from build123d import *

# Parameters (mm, degrees)
SKETCH1_R           = 25
SKETCH1_W           = 5
SKETCH1_H           = 10
SKETCH1_W_2         = 6
SKETCH1_H_2         = 8
BOSS_EXTRUDE1_DEPTH = 5


with BuildPart() as part:
    # Sketch1 → Boss-Extrude1 (new body)
    with BuildSketch(Plane.XY):
        with BuildLine():
            Line((-85, 10), (-85, 55))
            ThreePointArc((-85, 55), (-82.071067812, 62.071067812), (-75, 65))
            Line((-75, 65), (75, 65))
            ThreePointArc((75, 65), (82.071067812, 62.071067812), (85, 55))
            Line((85, 55), (85, 10))
            ThreePointArc((85, 10), (82.071067812, 2.928932188), (75, 0))
            Line((75, 0), (70, 0))
            ThreePointArc((70, 0), (40, -30), (10, 0))
            ThreePointArc((10, 0), (0, 10), (-10, 0))
            ThreePointArc((-10, 0), (-40, -30), (-70, 0))
            Line((-70, 0), (-75, 0))
            ThreePointArc((-75, 0), (-82.071067812, 2.928932188), (-85, 10))
        make_face()
        with Locations((-40, 0)):
            Circle(SKETCH1_R, mode=Mode.SUBTRACT)
        with Locations((40, 0)):
            Circle(SKETCH1_R, mode=Mode.SUBTRACT)
        with Locations((77.5, 17.5)):
            Rectangle(SKETCH1_W, SKETCH1_H, mode=Mode.SUBTRACT)
        with Locations((-77.5, 17.5)):
            Rectangle(SKETCH1_W, SKETCH1_H, mode=Mode.SUBTRACT)
        with Locations((-43, 42.5)):
            Rectangle(SKETCH1_W_2, SKETCH1_H_2, mode=Mode.SUBTRACT)
        with Locations((43, 42.5)):
            Rectangle(SKETCH1_W_2, SKETCH1_H_2, mode=Mode.SUBTRACT)
    extrude(amount=BOSS_EXTRUDE1_DEPTH)


solid = part.part
Geometry check sheet. Reference: the model listing, model coordinates, mm. A direction names the side the tool comes from. Round coordinates to 2 decimals unless told otherwise and drop trailing zeros. Order: outer loops, then holes, each group sorted by start corner. A loop starts at its lowest first (then second) coordinate and runs counter-clockwise, first axis right, second up. Notation, with made-up numbers: M 60,2 L 83,2 A17 ccw 83,25 Z; hole C -1,-5 d11. An arc over 180 degrees is marked long. Answer in a Markdown table with one row per item. Add a question column.
Item 1: Material ranges on L1, parallel to X at y = 45, z = 4.2; L2, parallel to X at y = -6, z = 4.6; L3, parallel to X at y = 1, z = 2.95, recorded low to high. Write a range as [from, to].
Item 2: Sectioned sample at A-A, the plane z = 3.25. State how many separate pieces and enclosed holes the cut face has, plus the area to 3 significant figures.
Item 3: Sectioned sample at C-C, the plane x = -60. Enter the section's corners in (y, z), plus the area to 3 significant figures.
Item 4: Depth check by flat-ended pin: pin 1 Ø2 at (x, z) = (-35.5, 4) entering from -Y; pin 2 Ø5 at (x, y) = (-66.5, -19) entering from -Z; pin 3 Ø2.5 at (x, z) = (76.5, 1.5) entering from -Y; pin 4 Ø1.5 at (x, z) = (-77.5, 2) entering from +Y. Enter the tip coordinate at first touch or a pass-through.
Item 5: Draft check along X on faces 3 (the face through (-82.15, 61.99, 2.46)), 4 (the face through (-1, 65, 2)), 5 (the face through (-80, 17, 2)). Enter one of: released by +X, released by -X, zero draft, split by the parting line, or undercut.
Item 6: Sectioned sample at D-D, the plane y = -11.5. Enter the section's corners in (x, z).
Item 7: Sectioned sample at B-B, the plane y = -23. Enter the section's corners in (x, z), plus the area to 3 significant figures.
Item 8: Set-up check for faces 1 (the face through (40.66, -29.993, 2.465)), 2 (the face through (75, 17, 2)): record each of +Z, -Z, +X, -X, +Y, -Y from which the full face is reachable in a straight line by a thin tool's end or side.
Filled in:
| question | item | result |
|---|---|---|
| 1 | L1 | x = [-85, -46], [-40, 40], [46, 85] |
| 1 | L2 | x = [-69.39, -64.27], [-15.73, -10.61], [10.61, 15.73], [64.27, 69.39] |
| 1 | L3 | x = [-79.36, -64.98], [-15.02, -9.95], [9.95, 15.02], [64.98, 79.36] |
| 2 | separate pieces | 1 |
| 2 | enclosed holes | 6 |
| 2 | area | 9,510 mm² |
| 3 | outline | M -22.36,0 L -15,0 L -15,5 L -22.36,5 Z; M 15,0 L 65,0 L 65,5 L 15,5 Z |
| 3 | area | 287 mm² |
| 4 | pin 1 | stops at y = -29.8 |
| 4 | pin 2 | passes through |
| 4 | pin 3 | stops at y = 0 |
| 4 | pin 4 | stops at y = 64.85 |
| 5 | face 3 | released by -X |
| 5 | face 4 | zero draft |
| 5 | face 5 | undercut |
| 6 | outline | M -67.71,0 L -62.2,0 L -62.2,5 L -67.71,5 Z; M -17.8,0 L -12.29,0 L -12.29,5 L -17.8,5 Z; M 12.29,0 L 17.8,0 L 17.8,5 L 12.29,5 Z; M 62.2,0 L 67.71,0 L 67.71,5 L 62.2,5 Z |
| 7 | outline | M -59.26,0 L -49.8,0 L -49.8,5 L -59.26,5 Z; M -30.2,0 L -20.74,0 L -20.74,5 L -30.2,5 Z; M 20.74,0 L 30.2,0 L 30.2,5 L 20.74,5 Z; M 49.8,0 L 59.26,0 L 59.26,5 L 49.8,5 Z |
| 7 | area | 189 mm² |
| 8 | face 1 | +Z, -Z, -Y |
| 8 | face 2 | +Z, -Z |
